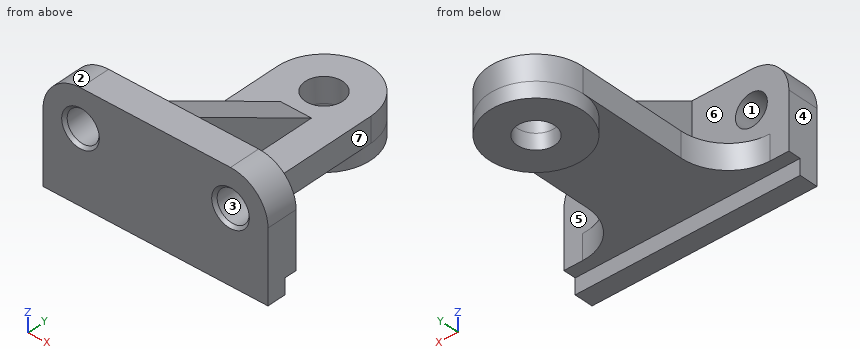
```python
from build123d import *
from build123d.topology import SkipClean

# Parameters (mm, degrees)
SKETCH1_W                    = 72
SKETCH1_H                    = 35
BOSS_EXTRUDE1_DEPTH          = 10
FILLET1_R                    = 12
CUT_EXTRUDE1_DEPTH           = 42.258332492
CUT_EXTRUDE1_DEPTH_BACK      = 42.258332492
SKETCH2_W                    = 5
SKETCH2_H                    = 4
M12_TAPPED_HOLE1_D           = 10.2
M12_TAPPED_HOLE1_CSINK_D     = 12.05
M12_TAPPED_HOLE1_CSINK_ANGLE = 90
SKETCH6_R                    = 6
BOSS_EXTRUDE2_DEPTH          = 8
FILLET2_R                    = 15
BOSS_EXTRUDE3_START          = 5
SKETCH7_R                    = 15
SKETCH7_R_2                  = 6
BOSS_EXTRUDE3_DEPTH          = 5
RIB5_START                   = -5
RIB5_DEPTH                   = 10


# Read off the part's stored shape, not the designer's step: Rib5
with BuildPart() as part:
    # Sketch1 → Boss-Extrude1 (new body)
    with BuildSketch(Plane(origin=(0, 0, 0), x_dir=(1, 0, 0), z_dir=(0, 1, 0))):
        Rectangle(SKETCH1_W, SKETCH1_H)
    extrude(amount=BOSS_EXTRUDE1_DEPTH)

    # Fillet1
    fillet1_edges = [part.edges().sort_by_distance(p)[0] for p in [
        (36, 5, 17.5),
        (-36, 5, 17.5),
    ]]
    fillet(fillet1_edges, radius=FILLET1_R)

    # Sketch2 → Cut-Extrude1 (cut, two sides: drawn at the far end of the back side and taken through both)
    with BuildSketch(Plane(origin=(0, 0, 0), x_dir=(0, 0, -1), z_dir=(1, 0, 0)).offset(-CUT_EXTRUDE1_DEPTH_BACK)):
        with Locations((15, 8)):
            Rectangle(SKETCH2_W, SKETCH2_H)
    extrude(amount=CUT_EXTRUDE1_DEPTH + CUT_EXTRUDE1_DEPTH_BACK, mode=Mode.SUBTRACT)

    # M12 Tapped Hole1 (through all)
    with Locations(Plane.XZ):
        with Locations((-24, 5.5), (24, 5.5)):
            CounterSinkHole(M12_TAPPED_HOLE1_D / 2, M12_TAPPED_HOLE1_CSINK_D / 2, counter_sink_angle=M12_TAPPED_HOLE1_CSINK_ANGLE)

    # Sketch6 → Boss-Extrude2 (add)
    with BuildSketch(Plane(origin=(0, 0, -12.5), x_dir=(-1, 0, 0), z_dir=(0, 0, -1))):
        with BuildLine():
            Line((15, 10), (-15, 10))
            Line((-15, 10), (-15, 60))
            ThreePointArc((-15, 60), (0, 75), (15, 60))
            Line((15, 60), (15, 10))
        make_face()
        with Locations((0, 60)):
            Circle(SKETCH6_R, mode=Mode.SUBTRACT)
    extrude(amount=-BOSS_EXTRUDE2_DEPTH)

    # Fillet2
    fillet2_edges = [part.edges().sort_by_distance(p)[0] for p in [
        (-15, 10, -8.5),
        (15, 10, -8.5),
    ]]
    fillet(fillet2_edges, radius=FILLET2_R)

    # Sketch7 → Boss-Extrude3 (add)
    with SkipClean():  # the faces are left unmerged after this step: merging them gives an invalid solid
        with BuildSketch(Plane(origin=(0, 0, -12.5), x_dir=(-1, 0, 0), z_dir=(0, 0, -1)).offset(BOSS_EXTRUDE3_START)):
            with Locations((0, 60)):
                Circle(SKETCH7_R)
            with Locations((0, 60)):
                Circle(SKETCH7_R_2, mode=Mode.SUBTRACT)
        extrude(amount=-BOSS_EXTRUDE3_DEPTH)

    # Rib5 outline → Rib5 (add)
    with SkipClean():  # the faces are left unmerged after this step: merging them gives an invalid solid
        with BuildSketch(Plane(origin=(0, 0, 0), x_dir=(0, 0, -1), z_dir=(1, 0, 0)).offset(RIB5_START)):
            Polygon((4.5, 50), (-17.5, 10), (4.5, 10), align=None)
        extrude(amount=RIB5_DEPTH)


solid = part.part
```
Input: part model. Units: mm. Frame: model coordinates. Face numbers are marked on the shaded views. A direction names the side the tool comes from. Round coordinates to 2 decimals unless told otherwise and drop trailing zeros. Loops run counter-clockwise (first coordinate to the right, second up) from the corner with the lowest first, then second, coordinate; pieces in that order, holes last. Notation, with made-up numbers: (36, 3) - (54, 3) arc R20 ccw to (54, 11) - close; hole circle Ø4 at (59.5, 37). An arc over 180 degrees is marked (long way). One line per item, written item: value. Start each with the question number.
(1) Access query for the marked faces 5, 6 and 7. Directions: +Z, -Z, +X, -X, +Y, -Y. A direction counts if a zero-diameter tool reaches every point of the face in a straight line with its end or side. Return the directions, or none.
(2) Section B-B, the plane z = -5.5. Return loops of the section in (x, y).
(3) Contact query for flat-ended pins moving along their axis: P1, Ø11.5, axis at x = 24, z = 5.5, coming from the -Y side (3 decimals); P2, Ø16.5, axis at x = -24, z = 5.5, coming from the +Y side; P3, Ø10, axis at x = -3.5, y = 22, coming from the +Z side; P4, Ø8, axis at x = -22.5, y = 61.5, coming from the -Z side. Output: stop coordinate, or through.
(4) Section C-C, the plane z = -14.5. Return loops of the section in (x, y).
(5) Ray query, line 1 (Y direction, x = 0, z = -10); line 2 (X direction, y = 3, z = 5); line 3 (Z direction, x = -10, y = 43.5). Return the intervals inside material, ascending. Write a range as [from, to].
(6) Section A-A, the plane x = 0. Return loops of the section in (y, z), plus the area to 3 significant figures.
(7) Section D-D, the plane y = 13. Return loops of the section in (x, z), plus the area to 4 significant figures.
(8) Draft query along Z for the marked faces 1, 2, 3 and 4. Return one class per face: +Z half, -Z half, draft (parallel to the pull), parting line (faces both ways), or undercut.
Results below:
1. face 5: +Z, +X, +Y
1. face 6: +Z, -X, +Y
1. face 7: +Z, -Z, +X, +Y
2. outline: (-36, 0) - (36, 0) - (36, 10) - (30, 10) arc R15 cw to (15, 25) - (15, 60) arc R15 ccw to (-15, 60) - (-15, 25) arc R15 cw to (-30, 10) - (-36, 10) - close; hole circle Ø12 at (0, 60)
3. P1: y = 0.275
3. P2: y = 10
3. P3: z = 13.65
3. P4: through
4. outline: (-36, 0) - (36, 0) - (36, 6) - (-36, 6) - close; circle Ø30 at (0, 60); hole circle Ø12 at (0, 60)
5. line 1: [0, 54], [66, 75]
5. line 2: [-36, -29.08], [-18.92, 18.92], [29.08, 36]
5. line 3: [-12.5, -4.5]
6. outline: (0, -17.5) - (6, -17.5) - (6, -12.5) - (45, -12.5) - (45, -17.5) - (54, -17.5) - (54, -4.5) - (50, -4.5) - (10, 17.5) - (0, 17.5) - close; (66, -17.5) - (75, -17.5) - (75, -4.5) - (66, -4.5) - close
6. area: 1,280 mm^2
7. outline: (-21, -12.5) - (21, -12.5) - (21, -4.5) - (5, -4.5) - (5, 15.85) - (-5, 15.85) - (-5, -4.5) - (-21, -4.5) - close
7. area: 539.5 mm^2
8. face 1: undercut
8. face 2: +Z half
8. face 3: undercut
8. face 4: draft
